Build history of the part. All positions in model axes, mm. A direction names the side the tool comes from. Coordinates: 2 decimals unless noted, no trailing zeros. Write each loop counter-clockwise with the first axis right and the second up, starting at its lowest first coordinate (ties: lowest second). Pieces come first, ordered by that corner, then holes.
from build123d import *

# Parameters (mm, degrees)
CROQUIS1_R              = 12.5
SALIENTE_EXTRUIR1_DEPTH = 54
CROQUIS2_R              = 15
SALIENTE_EXTRUIR2_DEPTH = 2.5
CROQUIS3_R              = 3.75
CORTAR_EXTRUIR2_DEPTH   = 2.5
CROQUIS5_R              = 1.5
CORTAR_EXTRUIR3_DEPTH   = 2.5
CROQUIS9_R              = 1.5
CORTAR_EXTRUIR5_DEPTH   = 2.5
SALIENTE_EXTRUIR3_DEPTH = 2.5
CROQUIS11_R             = 12.8
CORTAR_EXTRUIR6_DEPTH   = 54
CROQUIS12_R             = 1.7
CORTAR_EXTRUIR7_DEPTH   = 2.5
CROQUIS16_R             = 1.7
CORTAR_EXTRUIR8_DEPTH   = 2.5
CROQUIS17_R             = 1.7
CORTAR_EXTRUIR9_DEPTH   = 2.5


with BuildPart() as part:
    # Croquis1 → Saliente-Extruir1 (new body)
    with BuildSketch(Plane.XY):
        with BuildLine():
            Line((-5.119897429, -1.25), (-15, -1.25))
            Line((-15, -1.25), (-15, 1.25))
            Line((-15, 1.25), (15, 1.25))
            Line((15, 1.25), (15, -1.25))
            Line((15, -1.25), (5.119897429, -1.25))
            Line((5.119897429, -1.25), (5.119897429, -13.25))
            Line((5.119897429, -13.25), (5.119897429, -16.650828027))
            ThreePointArc((5.119897429, -16.650828027), (0, -45.75), (-5.119897429, -16.650828027))
            Line((-5.119897429, -16.650828027), (-5.119897429, -13.25))
            Line((-5.119897429, -13.25), (-5.119897429, -1.25))
        make_face()
        with Locations((0, -30.75)):
            Circle(CROQUIS1_R, mode=Mode.SUBTRACT)
    extrude(amount=SALIENTE_EXTRUIR1_DEPTH)

    # Croquis2 → Saliente-Extruir2 (add)
    with BuildSketch(Plane(origin=(0, 0, 0), x_dir=(-1, 0, 0), z_dir=(0, 0, -1))):
        with Locations((0, -30.75)):
            Circle(CROQUIS2_R)
    extrude(amount=SALIENTE_EXTRUIR2_DEPTH)

    # Croquis3 → Cortar-Extruir2 (cut)
    with BuildSketch(Plane(origin=(0, 0, -2.5), x_dir=(-1, 0, 0), z_dir=(0, 0, -1))):
        with Locations((0, -30.75)):
            Circle(CROQUIS3_R)
    extrude(amount=-CORTAR_EXTRUIR2_DEPTH, mode=Mode.SUBTRACT)

    # Croquis5 → Cortar-Extruir3 (cut)
    with BuildSketch(Plane(origin=(0, 0, -2.5), x_dir=(-1, 0, 0), z_dir=(0, 0, -1))):
        with Locations((0, -22.25)):
            Circle(CROQUIS5_R)
        with Locations((0, -39.25)):
            Circle(CROQUIS5_R)
    extrude(amount=-CORTAR_EXTRUIR3_DEPTH, mode=Mode.SUBTRACT)

    # Croquis9 → Cortar-Extruir5 (cut)
    with BuildSketch(Plane(origin=(0, 1.25, 0), x_dir=(1, 0, 0), z_dir=(0, 1, 0))):
        with Locations((-11.25, -50.625)):
            Circle(CROQUIS9_R)
        with Locations((-11.25, -3.375)):
            Circle(CROQUIS9_R)
        with Locations((11.25, -50.625)):
            Circle(CROQUIS9_R)
        with Locations((11.25, -3.375)):
            Circle(CROQUIS9_R)
    extrude(amount=-CORTAR_EXTRUIR5_DEPTH, mode=Mode.SUBTRACT)

    # Croquis10 → Saliente-Extruir3 (add)
    with BuildSketch(Plane(origin=(0, 0, 0), x_dir=(-1, 0, 0), z_dir=(0, 0, -1))):
        with BuildLine():
            Line((-15, 1.25), (15, 1.25))
            Line((15, 1.25), (15, -1.25))
            Line((15, -1.25), (5.119897429, -1.25))
            Line((5.119897429, -1.25), (5.119897429, -16.650828027))
            ThreePointArc((5.119897429, -16.650828027), (0, -15.75), (-5.119897429, -16.650828027))
            Line((-5.119897429, -16.650828027), (-5.119897429, -1.25))
            Line((-5.119897429, -1.25), (-15, -1.25))
            Line((-15, -1.25), (-15, 1.25))
        make_face()
    extrude(amount=SALIENTE_EXTRUIR3_DEPTH)

    # Croquis11 → Cortar-Extruir6 (cut)
    with BuildSketch(Plane.XY.offset(54)):
        with Locations((0, -30.75)):
            Circle(CROQUIS11_R)
    extrude(amount=-CORTAR_EXTRUIR6_DEPTH, mode=Mode.SUBTRACT)

    # Croquis12 → Cortar-Extruir7 (cut)
    with BuildSketch(Plane(origin=(0, 0, -2.5), x_dir=(-1, 0, 0), z_dir=(0, 0, -1))):
        with Locations((0, -22.25)):
            Circle(CROQUIS12_R)
        with Locations((0, -39.25)):
            Circle(CROQUIS12_R)
    extrude(amount=-CORTAR_EXTRUIR7_DEPTH, mode=Mode.SUBTRACT)

    # Croquis16 → Cortar-Extruir8 (cut)
    with BuildSketch(Plane(origin=(0, 1.25, 0), x_dir=(1, 0, 0), z_dir=(0, 1, 0))):
        with Locations((-11.25, -3.375)):
            Circle(CROQUIS16_R)
    extrude(amount=-CORTAR_EXTRUIR8_DEPTH, mode=Mode.SUBTRACT)

    # Croquis17 → Cortar-Extruir9 (cut)
    with BuildSketch(Plane(origin=(0, 1.25, 0), x_dir=(1, 0, 0), z_dir=(0, 1, 0))):
        with Locations((-11.25, -3.375)):
            Circle(CROQUIS17_R)
        with Locations((11.25, -3.375)):
            Circle(CROQUIS17_R)
        with Locations((-11.25, -50.625)):
            Circle(CROQUIS17_R)
        with Locations((11.25, -50.625)):
            Circle(CROQUIS17_R)
    extrude(amount=-CORTAR_EXTRUIR9_DEPTH, mode=Mode.SUBTRACT)


solid = part.part
(1) Probe L1, parallel to Z at x = 11.25, y = -0.1 (3 decimals); L2, parallel to Y at x = 0, z = -1; L3, parallel to Y at x = -11.5, z = 33.5. List the from-to ranges inside material, lowest first.
(2) Slice it at A-A, the plane z = 19.5. List the corners of the cut face in (x, y).
(3) Slice it at B-B, the plane y = -30.75. List the corners of the cut face in (x, z), and give its area (3 significant figures).
(4) Slice it at D-D, the plane x = -7. List the corners of the cut face in (y, z).
(5) 3-axis set-ups, long thin cutter, end or side, ignore diameter. For faces 5 (the cylindrical face through (-1.67, -18.06, 27.38)), 6 (the flat face through (-5.12, -9, 26)), 7 (the flat face through (5.12, -9, 26)), 8 (the cylindrical face through (12.034, 0.018, 52.133)): which of +Z, -Z, +X, -X, +Y, -Y reach the whole face in a straight line?
(6) Flat gauge pins, fed straight in: P1, Ø2, axis at x = -11.25, z = 50.625, coming from the -Y side; P2, Ø7.5, axis at x = 1, y = -34, coming from the +Z side; P3, Ø2.5, axis at x = -11.25, z = 3.375, coming from the +Y side; P4, Ø10, axis at x = 0, y = -30.75, coming from the -Z side. Where does each tip first touch, or does it go through?
(7) Slice it at C-C, the plane x = 1. List the corners of the cut face in (y, z).
(8) Two-plate mould, pull along Y, no slides. Class faces 1 (the flat face through (0, 1.25, 26)), 2 (the cylindrical face through (0.221, -20.564, -1.268)), 3 (the flat face through (-3, -28, 0)), 4 (the cylindrical face through (-10.466, 0.018, 52.133)): pulls with the +Y half, pulls with the -Y half, needs draft (parallel to the pull), parting line crosses it, or undercut.
Results:
1. L1: z = -2.5 to 1.675, 5.075 to 48.925, 52.325 to 54
1. L2: y = -45.75 to -40.95, -37.55 to -34.5, -27 to -23.95, -20.55 to 1.25
1. L3: y = -40.38 to -36.37, -25.13 to -21.12, -1.25 to 1.25
2. outline: (-15, -1.25) - (-5.12, -1.25) - (-5.12, -16.65) arc R15 ccw (long way) to (5.12, -16.65) - (5.12, -1.25) - (15, -1.25) - (15, 1.25) - (-15, 1.25) - close; hole circle Ø25.6 at (0, -30.75)
3. outline: (-15, -2.5) - (-3.75, -2.5) - (-3.75, 0) - (-12.8, 0) - (-12.8, 54) - (-15, 54) - close; (3.75, -2.5) - (15, -2.5) - (15, 54) - (12.8, 54) - (12.8, 0) - (3.75, 0) - close
3. area: 294 mm2
4. outline: (-44.02, -2.5) - (-17.48, -2.5) - (-17.48, 54) - (-20.03, 54) - (-20.03, 0) - (-41.47, 0) - (-41.47, 54) - (-44.02, 54) - close; (-1.25, -2.5) - (1.25, -2.5) - (1.25, 54) - (-1.25, 54) - close
5. face 5: +Z
5. face 6: +Z, -Z, -X
5. face 7: +Z, -Z, +X
5. face 8: +Y
6. P1: stops at y = -41.7
6. P2: stops at z = 0
6. P3: stops at y = -19.57
6. P4: stops at z = -2.5
7. outline: (-45.72, -2.5) - (-40.62, -2.5) - (-40.62, 0) - (-43.51, 0) - (-43.51, 54) - (-45.72, 54) - close; (-37.88, -2.5) - (-34.36, -2.5) - (-34.36, 0) - (-37.88, 0) - close; (-27.14, -2.5) - (-23.62, -2.5) - (-23.62, 0) - (-27.14, 0) - close; (-20.88, -2.5) - (1.25, -2.5) - (1.25, 54) - (-17.99, 54) - (-17.99, 0) - (-20.88, 0) - close
8. face 1: pulls with the +Y half
8. face 2: undercut
8. face 3: undercut
8. face 4: needs draft
